from build123d import *

# Parameters (mm, degrees)
FILLET1_R     = 4
CHAMFER1_SIZE = 1


with BuildPart() as part:
    # Sketch2 → Revolve1 (revolve)
    with BuildSketch(Plane(origin=(0, 0, 0), x_dir=(0, 0, -1), z_dir=(1, 0, 0)), mode=Mode.PRIVATE) as revolve1_sk:
        Polygon((10, 10), (10, 4.5), (15, 4.5), (15, 9.5), (25, 9.5), (25, -9.5), (15, -9.5), (15, -4.5), (10, -4.5), (10, -10), (5, -10), (5, 10), align=None)
    revolve(revolve1_sk.sketch.rotate(Axis((0, 38.551811756, 0), (0, -1, 0)), 180), axis=Axis((0, 38.551811756, 0), (0, -1, 0)))

    # Fillet1
    fillet1_edges = [part.edges().sort_by_distance(p)[0] for p in [
        (0, -9.5, -15),
        (0, -9.5, -25),
        (0, 9.5, -25),
    ]]
    fillet(fillet1_edges, radius=FILLET1_R)

    # Chamfer1
    chamfer1_edges = [part.edges().sort_by_distance(p)[0] for p in [
        (0, -10, -10),
        (0, 10, -10),
    ]]
    chamfer(chamfer1_edges, length=CHAMFER1_SIZE)


solid = part.part
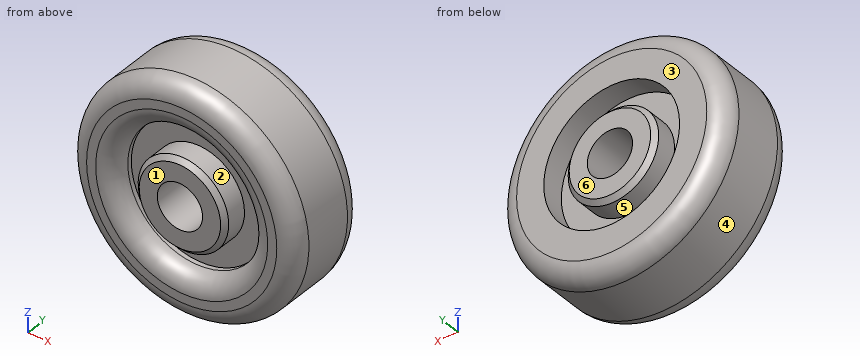
CAD build for the part. Positions are in the model's coordinates, mm. Face numbers are marked on the shaded views. A direction names the side the tool comes from. Round coordinates to 2 decimals unless told otherwise and drop trailing zeros. Write each loop counter-clockwise with the first axis right and the second up, starting at its lowest first coordinate (ties: lowest second). Pieces come first, ordered by that corner, then holes. Notation, with made-up numbers: (31, 0.25) -> (75, 0.25) arc R18 ccw to (75, 26.25) -> close; hole circle Ø2 at (-32, 19). An arc over 180 degrees is marked (long way). Answer as a JSON object with one key per item and string values.
(1) Pin check, flat tips, straight feed: P1, Ø24, axis at x = -6, z = -7.5, coming from the -Y side; P2, Ø1, axis at x = 7, y = -1, coming from the +Z side; P3, Ø6, axis at y = -2, z = -6, coming from the -X side; P4, Ø8, axis at y = -2, z = 16, coming from the +X side. Stop position of each tip, or through.
Reported:
{"P1": "stops at y = -10", "P2": "stops at z = 24.14", "P3": "stops at x = -24.82", "P4": "stops at x = 21.93"}
(2) Which spindle directions (+Z, -Z, +X, -X, +Y, -Y) get a long thin tool onto all of the face, cutting with end or side? Do the marked faces 1, 2 and 3. Say none if no direction does.
Reported:
{"face 1": "+Z, -Z, +X, -X, -Y", "face 2": "-Y", "face 3": "+Y"}
(3) Probe probe 1 along X at (y, z) = (-5.1, 0); probe 2 along X at (y, z) = (6.4, 0); probe 3 along X at (y, z) = (-0.25, 0). List the from-to ranges inside material, lowest first. Write a range as [from, to].
Reported:
{"probe 1": "x = [-25, -15], [-10, -5], [5, 10], [15, 25]", "probe 2": "x = [-24.9, -15], [-10, -5], [5, 10], [15, 24.9]", "probe 3": "x = [-25, -5], [5, 25]"}
(4) Two-plate mould, pull along X, no slides. Class the marked faces 4, 5 and 6: +X half, -X half, draft (parallel to the pull), parting line (faces both ways), or undercut.
Reported:
{"face 4": "parting line", "face 5": "undercut", "face 6": "draft"}
(5) Band-saw the part on C-C, the plane y = -6.5. List the corners of the cut face in (x, z), then the cut area to 3 significant figures.
Reported:
{"outline": "circle Ø49.75 at (0, 0); circle Ø20 at (0, 0); hole circle Ø30.25 at (0, 0); hole circle Ø10 at (0, 0)", "area": "1,460 mm^2"}
